Model file for the job. Use its own axes, mm. Coordinates: 2 decimals unless noted, no trailing zeros. Order: outer loops, then holes, each group sorted by start corner. A loop starts at its lowest first (then second) coordinate and runs counter-clockwise, first axis right, second up. Notation, with made-up numbers: (14, 89) -> (54, 89) arc R11 ccw to (54, 98) -> close; hole circle Ø11 at (58, -26). An arc over 180 degrees is marked (long way). Use CSV: the item, a comma, the result in double quotes. Start each with the question number.
(1) Probe L1, parallel to Y at x = 4, z = 1.6; L2, parallel to X at y = 0.2, z = 2.4; L3, parallel to Y at x = 3, z = 0.25. List the from-to ranges inside material, lowest first.
(2) Cut at B-B on y = 0. Write the cut outline in (x, z), plus the area to 3 significant figures.
(3) Cut at A-A on x = -4. Write the cut outline in (y, z), plus the area to 3 significant figures.
(4) Cut at C-C on z = 1.4. Write the cut outline in (x, y), plus the area to 3 significant figures.
```python
from build123d import *

# Parameters (mm, degrees)
SKETCH_1_W          = 16
SKETCH_1_H          = 6
EXTRUDE_1_DEPTH     = 3
SKETCH_2_R          = 1.5
CUT_EXTRUDE_1_DEPTH = 3


with BuildPart() as part:
    # ｽｹｯﾁ1 → ﾎﾞｽ - 押し出し1 (new body)
    with BuildSketch(Plane.XY):
        Rectangle(SKETCH_1_W, SKETCH_1_H)
    extrude(amount=EXTRUDE_1_DEPTH)

    # ｽｹｯﾁ2 → ｶｯﾄ - 押し出し1 (cut)
    with BuildSketch(Plane.XY.offset(3)):
        with Locations((-4, 0)):
            Circle(SKETCH_2_R)
        with Locations((4, 0)):
            Circle(SKETCH_2_R)
    extrude(amount=-CUT_EXTRUDE_1_DEPTH, mode=Mode.SUBTRACT)


solid = part.part
```
Outcome:
1,L1,"-3 to -1.5, 1.5 to 3"
1,L2,"-8 to -5.49, -2.51 to 2.51, 5.49 to 8"
1,L3,"-3 to -1.12, 1.12 to 3"
2,outline,"(-8, 0) -> (-5.5, 0) -> (-5.5, 3) -> (-8, 3) -> close; (-2.5, 0) -> (2.5, 0) -> (2.5, 3) -> (-2.5, 3) -> close; (5.5, 0) -> (8, 0) -> (8, 3) -> (5.5, 3) -> close"
2,area,"30.0 mm2"
3,outline,"(-3, 0) -> (-1.5, 0) -> (-1.5, 3) -> (-3, 3) -> close; (1.5, 0) -> (3, 0) -> (3, 3) -> (1.5, 3) -> close"
3,area,"9.00 mm2"
4,outline,"(-8, -3) -> (8, -3) -> (8, 3) -> (-8, 3) -> close; hole circle Ø3 at (-4, 0); hole circle Ø3 at (4, 0)"
4,area,"81.9 mm2"
